Check sheet for the modelled part. Datum: model origin and axes. Units: mm. A direction names the side the tool comes from. Coordinates: 2 decimals unless noted, no trailing zeros. Loops run counter-clockwise (first coordinate to the right, second up) from the corner with the lowest first, then second, coordinate; pieces in that order, holes last. Notation, with made-up numbers: M 70.25,-17.75 L 126.25,-17.75 A27 ccw 126.25,15.25 Z; hole C 48.5,12.5 d9. An arc over 180 degrees is marked long. Use CSV: the item, a comma, the result in double quotes. Start each with the question number.
(1) Draft check along Y on faces 1 (the flat face through (0, -37, 1)), 2 (the cylindrical face through (-13.392, -10.786, 12.779)), 3 (the flat face through (0, -18, 0)), 4 (the flat face through (-20.95, -29.13, 1.23)). Enter one of: pulls with the +Y half, pulls with the -Y half, needs draft (parallel to the pull), parting line crosses it, or undercut.
(2) Scan lines: line 1 (X direction, y = -3, z = 2.75); line 2 (Z direction, x = 11, y = -10); line 3 (Y direction, x = 15, z = 1). Record each from-to range of solid material in increasing order.
(3) Set-up check for faces 5 (the flat face through (21.231, -29.347, 1.232)), 6 (the flat face through (14, -13, 9)), 7 (the flat face through (-14, -13, 9)), 8 (the flat face through (0, -10, 2.5)): record each of +Z, -Z, +X, -X, +Y, -Y from which the full face is reachable in a straight line by a thin tool's end or side.
(4) Go/stop test with flat-tipped pins: pin 1 Ø6 at (x, y) = (-1.5, -34.5) entering from +Z; pin 2 Ø4 at (y, z) = (-17, 17.5) entering from -X; pin 3 Ø12 at (y, z) = (-29.5, 7) entering from -X. Record where each tip stops, or that it passes through.
(5) Section check C-C on y = -35. Record the cut outline in (x, z).
(6) Section check B-B on z = 15. Record the cut outline in (x, y), and give its area (3 significant figures).
(7) Section check D-D on y = -4. Record the cut outline in (x, z).
(8) Section check A-A on x = 7.5. Record the cut outline in (y, z), and give its area (3 significant figures).
from build123d import *

# Parameters (mm, degrees)
BOSS_EXTRUDE5_DEPTH     = 2.5
BOSS_EXTRUDE6_DEPTH     = 22
CUT_EXTRUDE2_DEPTH      = 72.527966559
CUT_EXTRUDE2_DEPTH_BACK = 72.527966559
SKETCH7_R               = 40


with BuildPart() as part:
    # Sketch2 → Boss-Extrude5 (new body)
    with BuildSketch(Plane.XY):
        Polygon((-14, 0), (14, 0), (14, -20), (40, -40), (-40, -40), (-14, -20), align=None)
        Polygon((-11, -21.477204492), (-31.17963416, -37), (31.17963416, -37), (11, -21.477204492), align=None, mode=Mode.SUBTRACT)
    extrude(amount=BOSS_EXTRUDE5_DEPTH)

    # Sketch6 → Boss-Extrude6 (add)
    with BuildSketch(Plane.XY.offset(2.5)):
        Polygon((-12.8, 0), (-14, 0), (-14, -21.477204492), (14, -21.477204492), (14, 0), (12.8, 0), (12.8, -20.277204492), (-12.8, -20.277204492), align=None)
    extrude(amount=BOSS_EXTRUDE6_DEPTH)

    # Sketch7 → Cut-Extrude2 (cut, two sides: drawn at the far end of the back side and taken through both)
    with BuildSketch(Plane.ZY.offset(14).offset(-CUT_EXTRUDE2_DEPTH_BACK)):
        with Locations((40, 18.522795508)):
            Circle(SKETCH7_R)
    extrude(amount=CUT_EXTRUDE2_DEPTH + CUT_EXTRUDE2_DEPTH_BACK, mode=Mode.SUBTRACT)


solid = part.part
Outcome:
1,face 1,"undercut"
1,face 2,"pulls with the +Y half"
1,face 3,"needs draft"
1,face 4,"undercut"
2,line 1,"x = -14 to -12.8, 12.8 to 14"
2,line 2,"z = 0 to 2.5"
2,line 3,"y = -40 to -37, -24.55 to -20.77"
3,face 5,"+Z, -Z"
3,face 6,"+Z, +X, +Y"
3,face 7,"+Z, -X, +Y"
3,face 8,"+Z, +Y"
4,pin 1,"stops at z = 2.5"
4,pin 2,"stops at x = -14"
4,pin 3,"stops at x = -31.51"
5,outline,"M -33.5,0 L -28.58,0 L -28.58,2.5 L -33.5,2.5 Z; M 28.58,0 L 33.5,0 L 33.5,2.5 L 28.58,2.5 Z"
6,outline,"M -14,-21.48 L 14,-21.48 L 14,-12.7 L 12.8,-12.7 L 12.8,-20.28 L -12.8,-20.28 L -12.8,-12.7 L -14,-12.7 Z"
6,area,"51.8 mm²"
7,outline,"M -14,0 L 14,0 L 14,6.94 L 12.8,6.94 L 12.8,2.5 L -12.8,2.5 L -12.8,6.94 L -14,6.94 Z"
8,outline,"M -40,0 L -37,0 L -37,2.5 L -40,2.5 Z; M -21.48,0 L 0,0 L 0,2.5 L -20.28,2.5 L -20.28,24.5 L -21.48,24.5 Z"
8,area,"87.6 mm²"
